```python
from build123d import *

# Parameters (mm, degrees)
SKETCH9_W               = 1.8
SKETCH9_H               = 5.8
BOSS_EXTRUDE8_DEPTH     = 4
BOSS_EXTRUDE8_2_DEPTH   = 4
BOSS_EXTRUDE8_3_DEPTH   = 4
BOSS_EXTRUDE8_4_DEPTH   = 4
BOSS_EXTRUDE8_5_DEPTH   = 4
BOSS_EXTRUDE8_6_DEPTH   = 4
SKETCH9_W_2             = 5.8
SKETCH9_H_2             = 1.8
BOSS_EXTRUDE8_7_DEPTH   = 4
BOSS_EXTRUDE8_8_DEPTH   = 4
BOSS_EXTRUDE8_9_DEPTH   = 4
BOSS_EXTRUDE5_DEPTH     = 19
BOSS_EXTRUDE6_DEPTH     = 2
BOSS_EXTRUDE11_DEPTH    = 1
CUT_EXTRUDE6_DEPTH      = 99.442876837
CUT_EXTRUDE6_DEPTH_BACK = 99.442876837
SKETCH18_W              = 19
SKETCH18_H              = 16
SKETCH19_W              = 24.4
SKETCH19_H              = 19
CUT_EXTRUDE8_DEPTH      = 99.442876837
CUT_EXTRUDE9_START      = -19
SKETCH10_W              = 10
SKETCH10_H              = 34
CUT_EXTRUDE9_DEPTH      = 19
FILLET3_R               = 4
FILLET4_R               = 5
FILLET5_R               = 3


with BuildPart() as part:
    # Sketch9 → Boss-Extrude8 (new body)
    with BuildSketch(Plane(origin=(0, 0, 0), x_dir=(1, 0, 0), z_dir=(0, 0, -1))):
        with Locations((-85, 30)):
            Rectangle(SKETCH9_W, SKETCH9_H)
    extrude(amount=BOSS_EXTRUDE8_DEPTH)



with BuildPart() as body_2:
    # Sketch9 → Boss-Extrude8 2 (new body)
    with BuildSketch(Plane(origin=(0, 0, 0), x_dir=(1, 0, 0), z_dir=(0, 0, -1))):
        with Locations((-85, 0)):
            Rectangle(SKETCH9_W, SKETCH9_H)
    extrude(amount=BOSS_EXTRUDE8_2_DEPTH)


with BuildPart() as body_3:
    # Sketch9 → Boss-Extrude8 3 (new body)
    with BuildSketch(Plane(origin=(0, 0, 0), x_dir=(1, 0, 0), z_dir=(0, 0, -1))):
        with Locations((-85, -30)):
            Rectangle(SKETCH9_W, SKETCH9_H)
    extrude(amount=BOSS_EXTRUDE8_3_DEPTH)


with BuildPart() as body_4:
    # Sketch9 → Boss-Extrude8 4 (new body)
    with BuildSketch(Plane(origin=(0, 0, 0), x_dir=(1, 0, 0), z_dir=(0, 0, -1))):
        with Locations((85, 30)):
            Rectangle(SKETCH9_W, SKETCH9_H)
    extrude(amount=BOSS_EXTRUDE8_4_DEPTH)


with BuildPart() as body_5:
    # Sketch9 → Boss-Extrude8 5 (new body)
    with BuildSketch(Plane(origin=(0, 0, 0), x_dir=(1, 0, 0), z_dir=(0, 0, -1))):
        with Locations((85, -30)):
            Rectangle(SKETCH9_W, SKETCH9_H)
    extrude(amount=BOSS_EXTRUDE8_5_DEPTH)


with BuildPart() as body_6:
    # Sketch9 → Boss-Extrude8 6 (new body)
    with BuildSketch(Plane(origin=(0, 0, 0), x_dir=(1, 0, 0), z_dir=(0, 0, -1))):
        with Locations((85, 0)):
            Rectangle(SKETCH9_W, SKETCH9_H)
    extrude(amount=BOSS_EXTRUDE8_6_DEPTH)


with BuildPart() as body_7:
    # Sketch9 → Boss-Extrude8 7 (new body)
    with BuildSketch(Plane(origin=(0, 0, 0), x_dir=(1, 0, 0), z_dir=(0, 0, -1))):
        with Locations((-64.5, 39)):
            Rectangle(SKETCH9_W_2, SKETCH9_H_2)
    extrude(amount=BOSS_EXTRUDE8_7_DEPTH)


with BuildPart() as body_8:
    # Sketch9 → Boss-Extrude8 8 (new body)
    with BuildSketch(Plane(origin=(0, 0, 0), x_dir=(1, 0, 0), z_dir=(0, 0, -1))):
        with Locations((0, 39)):
            Rectangle(SKETCH9_W_2, SKETCH9_H_2)
    extrude(amount=BOSS_EXTRUDE8_8_DEPTH)


with BuildPart() as body_9:
    # Sketch9 → Boss-Extrude8 9 (new body)
    with BuildSketch(Plane(origin=(0, 0, 0), x_dir=(1, 0, 0), z_dir=(0, 0, -1))):
        with Locations((64.5, 39)):
            Rectangle(SKETCH9_W_2, SKETCH9_H_2)
    extrude(amount=BOSS_EXTRUDE8_9_DEPTH)


with BuildPart() as part_1:
    add(part.part)

    add(body_2.part)  # Boss-Extrude5 merges body 2

    add(body_3.part)  # Boss-Extrude5 merges body 3

    add(body_4.part)  # Boss-Extrude5 merges body 4

    add(body_5.part)  # Boss-Extrude5 merges body 5

    add(body_6.part)  # Boss-Extrude5 merges body 6

    add(body_7.part)  # Boss-Extrude5 merges body 7

    add(body_8.part)  # Boss-Extrude5 merges body 8

    add(body_9.part)  # Boss-Extrude5 merges body 9
    # Sketch1 → Boss-Extrude5 (add)
    with BuildSketch(Plane.XY):
        Polygon((-87, 41), (-85, 41), (-85, -39), (85, -39), (85, 41), (87, 41), (87, -41), (-87, -41), align=None)
    extrude(amount=BOSS_EXTRUDE5_DEPTH)

    # Sketch7 → Boss-Extrude6 (add)
    with BuildSketch(Plane.XY.offset(19)):
        Polygon((-87, 41), (-77, 41), (-77, -31), (77, -31), (77, 41), (87, 41), (87, -41), (-87, -41), align=None)
    extrude(amount=BOSS_EXTRUDE6_DEPTH)

    # Sketch17 → Boss-Extrude11 (add)
    with BuildSketch(Plane.XY):
        Polygon((-84, 41), (-85, 41), (-85, -39), (85, -39), (85, 41), (84, 41), (84, -38), (-84, -38), align=None)
    extrude(amount=BOSS_EXTRUDE11_DEPTH)

    # Sketch18 → Cut-Extrude6 (cut, two sides: drawn at the far end of the back side and taken through both)
    with BuildSketch(Plane.ZY.offset(-CUT_EXTRUDE6_DEPTH_BACK)):
        with Locations((11.5, 25)):
            Rectangle(SKETCH18_W, SKETCH18_H)
        with Locations((11.5, 1)):
            Rectangle(SKETCH18_W, SKETCH18_H)
        with Locations((11.5, -23)):
            Rectangle(SKETCH18_W, SKETCH18_H)
    extrude(amount=CUT_EXTRUDE6_DEPTH + CUT_EXTRUDE6_DEPTH_BACK, mode=Mode.SUBTRACT)

    # Sketch19 → Cut-Extrude8 (cut, through all)
    with BuildSketch(Plane.XZ):
        with Locations((-64.8, 11.5)):
            Rectangle(SKETCH19_W, SKETCH19_H)
        with Locations((-32.4, 11.5)):
            Rectangle(SKETCH19_W, SKETCH19_H)
        with Locations((0, 11.5)):
            Rectangle(SKETCH19_W, SKETCH19_H)
        with Locations((32.4, 11.5)):
            Rectangle(SKETCH19_W, SKETCH19_H)
        with Locations((64.8, 11.5)):
            Rectangle(SKETCH19_W, SKETCH19_H)
    extrude(amount=CUT_EXTRUDE8_DEPTH, mode=Mode.SUBTRACT)

    # Sketch10 → Cut-Extrude9 (cut)
    with BuildSketch(Plane.XY.offset(21).offset(CUT_EXTRUDE9_START)):
        with Locations((82, -7)):
            Rectangle(SKETCH10_W, SKETCH10_H)
    extrude(amount=CUT_EXTRUDE9_DEPTH, mode=Mode.SUBTRACT)

    # Fillet3
    # the kernel refuses this fillet: 4 mm, written as the material it takes off along each edge
    with BuildSketch(Plane(origin=(77, 41, 9), x_dir=(0, -1, 0), z_dir=(0, 0, 1)), Plane(origin=(-77, 33, 9), x_dir=(0, 1, 0), z_dir=(0, 0, 1)), Plane(origin=(77, 17, 9), x_dir=(0, -1, 0), z_dir=(0, 0, 1)), Plane(origin=(-77, 17, 31), x_dir=(0, -1, 0), z_dir=(0, 0, -1)), Plane(origin=(-77, 9, 9), x_dir=(0, 1, 0), z_dir=(0, 0, 1)), Plane(origin=(-77, -7, 31), x_dir=(0, -1, 0), z_dir=(0, 0, -1)), Plane(origin=(-77, -15, 9), x_dir=(0, 1, 0), z_dir=(0, 0, 1)), Plane(origin=(-44.6, -31, 9), x_dir=(-1, 0, 0), z_dir=(0, 0, 1)), Plane(origin=(-12.2, -31, 9), x_dir=(-1, 0, 0), z_dir=(0, 0, 1)), Plane(origin=(20.2, -31, 9), x_dir=(-1, 0, 0), z_dir=(0, 0, 1)), Plane(origin=(52.6, -31, 9), x_dir=(-1, 0, 0), z_dir=(0, 0, 1)), Plane(origin=(77, 10, 9), x_dir=(1, 0, 0), z_dir=(0, 0, 1))) as fillet3_piece_1:
        with BuildLine():
            CenterArc((FILLET3_R, FILLET3_R), FILLET3_R, 180, 90)
            Line((0, FILLET3_R), (0, 0))
            Line((0, 0), (FILLET3_R, 0))
        make_face()
    extrude(amount=22, mode=Mode.SUBTRACT)
    with BuildSketch(Plane(origin=(-77, 41, 9), x_dir=(0, -1, 0), z_dir=(0, 0, 1)), Plane(origin=(77, 33, 31), x_dir=(1, 0, 0), z_dir=(0, 0, -1)), Plane(origin=(-77, -31, 9), x_dir=(0, -1, 0), z_dir=(0, 0, 1)), Plane(origin=(-52.6, -31, 31), x_dir=(0, -1, 0), z_dir=(0, 0, -1)), Plane(origin=(-20.2, -31, 31), x_dir=(0, -1, 0), z_dir=(0, 0, -1)), Plane(origin=(12.2, -31, 31), x_dir=(0, -1, 0), z_dir=(0, 0, -1)), Plane(origin=(44.6, -31, 31), x_dir=(0, -1, 0), z_dir=(0, 0, -1)), Plane(origin=(77, -31, 31), x_dir=(0, -1, 0), z_dir=(0, 0, -1))) as fillet3_piece_2:
        with BuildLine():
            CenterArc((FILLET3_R, -FILLET3_R), FILLET3_R, 90, 90)
            Line((0, -FILLET3_R), (0, 0))
            Line((0, 0), (FILLET3_R, 0))
        make_face()
    extrude(amount=22, mode=Mode.SUBTRACT)

    # Fillet4
    fillet4_edges = [part_1.edges().sort_by_distance(p)[0] for p in [
        (86, 17, 2),
        (-86, 17, 2),
        (86, 33, 2),
        (-86, 33, 2),
        (-86, -7, 2),
        (-86, 9, 2),
        (86, -31, 2),
        (-86, -31, 2),
        (-86, -15, 2),
        (-77, -40, 2),
        (-52.6, -40, 2),
        (-44.6, -40, 2),
        (-20.2, -40, 2),
        (-12.2, -40, 2),
        (12.2, -40, 2),
        (20.2, -40, 2),
        (44.6, -40, 2),
        (52.6, -40, 2),
        (77, -40, 2),
        (86, 10, 2),
    ]]
    fillet(fillet4_edges, radius=FILLET4_R)

    # Fillet5
    fillet5_edges = [part_1.edges().sort_by_distance(p)[0] for p in [
        (-87, 41, 10.5),
        (-87, -41, 10.5),
        (87, -41, 10.5),
        (87, 41, 10.5),
    ]]
    fillet(fillet5_edges, radius=FILLET5_R)


solid = part_1.part
```
Check sheet for the modelled part. Datum: model origin and axes. Units: mm. A direction names the side the tool comes from. Round coordinates to 2 decimals unless told otherwise and drop trailing zeros. Loops run counter-clockwise (first coordinate to the right, second up) from the corner with the lowest first, then second, coordinate; pieces in that order, holes last. Notation, with made-up numbers: (37.25, 23) - (87.25, 23) arc R13 cw to (87.25, 43) - close; hole circle Ø4 at (47, 46). An arc over 180 degrees is marked (long way). Answer as a JSON object with one key per item and string values. Group by question number.
Q1. Mould release check, pull along Z, two halves, no side actions. Record for faces 1 (the face through (-82, -11, 21)), 2 (the face through (85, 3.7, 1.3)), 3 (the face through (-77, 13, 20)): released by +Z, released by -Z, zero draft, split by the parting line, or undercut.
Q2. Scan lines: line 1 along X through (y, z) = (15, 8.5); line 2 along X through (y, z) = (-8, 12); line 3 along Y through (x, z) = (48, 17.75). Record each from-to range of solid material in increasing order. Write a range as [from, to].
Q3. Sectioned sample at C-C, the plane x = 48.6. Enter the section's corners in (y, z), plus the area to 3 significant figures.
Q4. Set-up check for faces 4 (the face through (-85.3, -15, 15.5)), 5 (the face through (16, -35, 19)), 6 (the face through (10.77, -40.01, 3.5)): record each of +Z, -Z, +X, -X, +Y, -Y from which the full face is reachable in a straight line by a thin tool's end or side.
Q5. Sectioned sample at B-B, the plane z = -1.75. Count the separate pieces of the cut face and the enclosed holes in it, plus the area to 3 significant figures.
Q6. Gauge pin test, flat ends, axial feed: P1, Ø2, axis at y = -38.5, z = -1.5, coming from the +X side; P2, Ø1.2, axis at x = 63.5, z = -2, coming from the -Y side; P3, Ø5, axis at x = -53.5, z = 17.5, coming from the +Y side (3 decimals); P4, Ø12, axis at x = -60.5, z = 7, coming from the -Y side. Record the tip position at first contact, or that the pin passes through.
Q7. Sectioned sample at A-A, the plane y = -23.5. Enter the section's corners in (x, z), plus the area to 3 significant figures.
Solution:
{
 "1": {"face 1": "released by +Z", "face 2": "undercut", "face 3": "zero draft"},
 "2": {"line 1": "x = [-87, -85], [85, 87]", "line 2": "x = [-87, -85]", "line 3": "y = [-41, -39]"},
 "3": {"outline": "(-41, 0) - (-38, 0) - (-38, 1) - (-39, 1) - (-39, 19) - (-31, 19) - (-31, 21) - (-41, 21) - close", "area": "59.0 mm²"},
 "4": {"face 4": "+Z, +X, -X", "face 5": "+Y", "face 6": "+Z, +Y, -Y"},
 "5": {"separate pieces": "9", "enclosed holes": "0", "area": "94.0 mm²"},
 "6": {"P1": "stops at x = 67.4", "P2": "stops at y = -39.9", "P3": "stops at y = -32.245", "P4": "stops at y = -41"},
 "7": {"outline": "(-87, 0) - (-84, 0) - (-84, 1) - (-85, 1) - (-85, 2) - (-87, 2) - close; (84, 0) - (87, 0) - (87, 2) - (85, 2) - (85, 1) - (84, 1) - close", "area": "10.0 mm²"}
}
